CAD build for the part. Positions are in the model's coordinates, mm. Face numbers are marked on the shaded views. A direction names the side the tool comes from. Give positions to 0.01 mm unless a question says otherwise; leave off trailing zeros. Write each loop counter-clockwise with the first axis right and the second up, starting at its lowest first coordinate (ties: lowest second). Pieces come first, ordered by that corner, then holes. Notation, with made-up numbers: (67, 24.25) - (84, 24.25) arc R27 ccw to (84, 56.25) - close; hole circle Ø7 at (40.25, 52). An arc over 180 degrees is marked (long way). Answer as a JSON object with one key per item and string values.
from build123d import *

# Parameters (mm, degrees)
SKETCH1_W                    = 86
SKETCH1_H                    = 86
BOSS_EXTRUDE1_DEPTH          = 82.721
SKETCH2_R                    = 36.575
CUT_EXTRUDE1_DEPTH           = 1.449994037
SKETCH3_R                    = 20.5
CUT_EXTRUDE2_DEPTH           = 61.5
SKETCH4_R                    = 18.5
CUT_EXTRUDE3_DEPTH           = 12.5
SKETCH5_R                    = 7.5
CUT_EXTRUDE4_DEPTH           = 438.22445056
CUT_EXTRUDE5_REACH           = 382.784
CUT_EXTRUDE5_END_RADIUS      = 20.5
SKETCH6_W                    = 14
SKETCH6_H                    = 50
F_7_0_7_DIAMETER_HOLE1_D     = 7
F_7_0_7_DIAMETER_HOLE1_DEPTH = 22
F_7_0_7_DIAMETER_HOLE2_D     = 7
F_7_0_7_DIAMETER_HOLE2_DEPTH = 25.000212861


with BuildPart() as part:
    # Sketch1 → Boss-Extrude1 (new body)
    with BuildSketch(Plane(origin=(0, 0, 0), x_dir=(-1, 0, 0), z_dir=(0, 0, -1))):
        with Locations((318.604600328, 194.58078929)):
            Rectangle(SKETCH1_W, SKETCH1_H)
    extrude(amount=-BOSS_EXTRUDE1_DEPTH)

    # Sketch2 → Cut-Extrude1 (cut)
    with BuildSketch(Plane.XY.offset(82.721)):
        with Locations(Location((-318.604600328, 194.58078929, 0), (0, 0, 180))):
            Circle(SKETCH2_R)
    extrude(amount=-CUT_EXTRUDE1_DEPTH, mode=Mode.SUBTRACT)

    # Sketch3 → Cut-Extrude2 (cut)
    with BuildSketch(Plane.XY.offset(81.271005963)):
        with Locations(Location((-318.604600328, 194.58078929, 0), (0, 0, 180))):
            Circle(SKETCH3_R)
    extrude(amount=-CUT_EXTRUDE2_DEPTH, mode=Mode.SUBTRACT)

    # Sketch4 → Cut-Extrude3 (cut)
    with BuildSketch(Plane(origin=(0, 0, 0), x_dir=(-1, 0, 0), z_dir=(0, 0, -1))):
        with Locations(Location((318.604600328, 194.58078929, 0), (0, 0, 180))):
            Circle(SKETCH4_R)
    extrude(amount=-CUT_EXTRUDE3_DEPTH, mode=Mode.SUBTRACT)

    # Sketch5 → Cut-Extrude4 (cut, through all)
    with BuildSketch(Plane.XY.offset(19.771005963)):
        with Locations((-318.604600328, 194.58078929)):
            Circle(SKETCH5_R)
    extrude(amount=-CUT_EXTRUDE4_DEPTH, mode=Mode.SUBTRACT)

    # Cut-Extrude5: up to this cylinder (the profile starts outside it)
    cut_extrude5_end = Plane(origin=(-318.604600328, 194.58078929, 44.930798), z_dir=(0, 0, 1)) * Cylinder(CUT_EXTRUDE5_END_RADIUS, 807.568, mode=Mode.PRIVATE)
    # Sketch6 → Cut-Extrude5 (cut, up to the surface)
    with BuildSketch(Plane(origin=(0, 237.58078929, 0), x_dir=(-1, 0, 0), z_dir=(0, 1, 0)), mode=Mode.PRIVATE) as cut_extrude5_sk1:
        with Locations((305.604600328, 44.930797937)):
            Rectangle(SKETCH6_W, SKETCH6_H)
    cut_extrude5_tool1 = extrude(cut_extrude5_sk1.sketch, amount=-CUT_EXTRUDE5_REACH, mode=Mode.PRIVATE) - cut_extrude5_end
    add(cut_extrude5_tool1.solids().sort_by_distance((-305.6046, 237.580789, 44.930798))[0], mode=Mode.SUBTRACT)

    # Ø7.0 (7) Diameter Hole1
    with Locations(Plane(origin=(0, 0, 0), x_dir=(-1, 0, 0), z_dir=(0, 0, -1))):
        with Locations((283.604600328, 159.58078929), (283.604600328, 229.58078929), (353.604600328, 159.58078929), (353.604600328, 229.58078929)):
            Hole(F_7_0_7_DIAMETER_HOLE1_D / 2, depth=F_7_0_7_DIAMETER_HOLE1_DEPTH)

    # Ø7.0 (7) Diameter Hole2
    with Locations(Plane.XY.offset(82.721)):
        with Locations((-283.249261269, 159.22545023), (-353.959939388, 229.936128349), (-283.249261269, 229.936128349), (-353.959939388, 159.22545023)):
            Hole(F_7_0_7_DIAMETER_HOLE2_D / 2, depth=F_7_0_7_DIAMETER_HOLE2_DEPTH)


solid = part.part
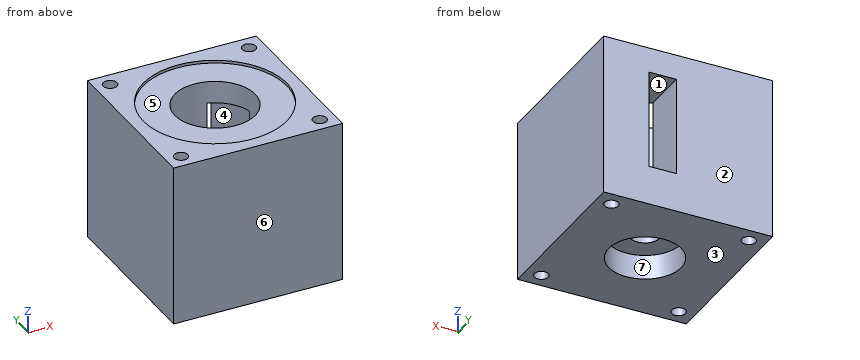
(1) 3-axis set-ups, long thin cutter, end or side, ignore diameter. For the marked faces 4, 5, 6 and 7: which of +Z, -Z, +X, -X, +Y, -Y reach the whole face in a straight line?
Answer key:
{"face 4": "+Y", "face 5": "+Z", "face 6": "+Z, -Z, +X, -X, -Y", "face 7": "-Z"}
(2) Flat gauge pins, fed straight in: P1, Ø4, axis at x = -309, y = 226, coming from the +Z side; P2, Ø3.5, axis at x = -284.5, y = 160.5, coming from the -Z side; P3, Ø1.5, axis at x = -310, z = 66, coming from the +Y side. Where does each tip first touch, or does it go through?
Answer key:
{"P1": "stops at z = 81.27", "P2": "stops at z = 22", "P3": "stops at y = 176.34"}
(3) Saw through at C-C, the plane x = -319. Give the cut face in (y, z), and give its area (3 significant figures).
Answer key:
{"outline": "(151.58, 0) - (176.09, 0) - (176.09, 12.5) - (187.09, 12.5) - (187.09, 19.77) - (174.08, 19.77) - (174.08, 81.27) - (158.01, 81.27) - (158.01, 82.72) - (151.58, 82.72) - close; (202.07, 12.5) - (213.08, 12.5) - (213.08, 0) - (237.58, 0) - (237.58, 82.72) - (231.15, 82.72) - (231.15, 81.27) - (215.08, 81.27) - (215.08, 19.77) - (202.07, 19.77) - close", "area": "3,920 mm²"}
(4) Saw through at B-B, the plane z = 14. Give the cut face in (x, y), and give its area (3 significant figures).
Answer key:
{"outline": "(-361.6, 151.58) - (-275.6, 151.58) - (-275.6, 237.58) - (-361.6, 237.58) - close; hole circle Ø7 at (-353.6, 159.58); hole circle Ø7 at (-353.6, 229.58); hole circle Ø15 at (-318.6, 194.58); hole circle Ø7 at (-283.6, 159.58); hole circle Ø7 at (-283.6, 229.58)", "area": "7,070 mm²"}
(5) Saw through at A-A, the plane y = 190. Give the cut face in (x, z), and give its area (3 significant figures).
Answer key:
{"outline": "(-361.6, 0) - (-336.53, 0) - (-336.53, 12.5) - (-324.54, 12.5) - (-324.54, 19.77) - (-338.59, 19.77) - (-338.59, 81.27) - (-354.89, 81.27) - (-354.89, 82.72) - (-361.6, 82.72) - close; (-312.67, 12.5) - (-300.68, 12.5) - (-300.68, 0) - (-275.6, 0) - (-275.6, 82.72) - (-282.32, 82.72) - (-282.32, 81.27) - (-298.62, 81.27) - (-298.62, 19.77) - (-312.67, 19.77) - close", "area": "4,020 mm²"}
(6) Saw through at D-D, the plane z = 25. Give the cut face in (x, y), and give its area (3 significant figures).
Answer key:
{"outline": "(-361.6, 151.58) - (-275.6, 151.58) - (-275.6, 237.58) - (-298.6, 237.58) - (-298.6, 199.08) arc R20.5 cw (long way) to (-312.6, 214.18) - (-312.6, 237.58) - (-361.6, 237.58) - close", "area": "5,680 mm²"}
(7) Pull direction Z, two halves, no side cores. Call the marked faces 1, 2 and 3: pulls with the +Z half, pulls with the -Z half, needs draft (parallel to the pull), parting line crosses it, or undercut.
Answer key:
{"face 1": "undercut", "face 2": "needs draft", "face 3": "pulls with the -Z half"}
(8) Probe L1, parallel to X at y = 157.5, z = 18.5; L2, parallel to X at y = 217, z = 64; L3, parallel to Z at x = -333, y = 165. List the from-to ranges inside material, lowest first. Write a range as [from, to].
Answer key:
{"L1": "x = [-361.6, -356.42], [-350.79, -286.42], [-280.79, -275.6]", "L2": "x = [-361.6, -312.6], [-298.6, -275.6]", "L3": "z = [0, 81.27]"}
